Check sheet for the modelled part. Datum: model origin and axes. Units: mm. A direction names the side the tool comes from. Coordinates: 2 decimals unless noted, no trailing zeros. Order: outer loops, then holes, each group sorted by start corner. A loop starts at its lowest first (then second) coordinate and runs counter-clockwise, first axis right, second up. Notation, with made-up numbers: M 66,69 L 122,69 A31 ccw 122,102 Z; hole C -6,5 d8. An arc over 180 degrees is marked long. Answer in a Markdown table with one row per item. Add a question column.
from build123d import *

# Parameters (mm, degrees)
AUFSATZ_LINEAR_AUSTRAGEN1_DEPTH = 1566.7
SCHNITT_LINEAR_AUSTRAGEN1_REACH = 1704.359
FASE1_SIZE2                     = 30
FASE1_SIZE                      = 22
VERRUNDUNG1_R                   = 10
SKIZZE4_R                       = 14.488887394336269
AUFSATZ_LINEAR_AUSTRAGEN3_DEPTH = 30
AUFSATZ_LINEAR_AUSTRAGEN7_REACH = 1402.712
LINEARES_MUSTER2_COUNT          = 2
LINEARES_MUSTER2_PITCH          = 770.0000000000005


with BuildPart() as part:
    # Skizze1 → Aufsatz-Linear austragen1 (new body)
    with BuildSketch(Plane.XY):
        Polygon((650.3604764885325, 174.22108378429925), (650.3604764885325, 144.22108378429925), (227.86047648853256, 257.42961758644554), (72.86047648853256, 257.42961758644554), (-349.6395235114674, 144.22108378429914), (-349.6395235114674, 174.2210837842995), (72.86047648853253, 287.42961758644606), (227.8604764885318, 287.42961758644606), align=None)
    extrude(amount=AUFSATZ_LINEAR_AUSTRAGEN1_DEPTH)

    # Skizze2 → Schnitt-Linear austragen1 (cut, up to next)
    with BuildSketch(Plane(origin=(0, 287.42961758644606, 0), x_dir=(1, 0, 0), z_dir=(0, 1, 0)), mode=Mode.PRIVATE) as schnitt_linear_austragen1_sk1:
        Polygon((145.36047648853253, -360), (-289.47952351146745, -360.00000000000006), (-289.47952351146733, -1160.0000000000002), (145.36047648853264, -1160.0000000000005), align=None)
    schnitt_linear_austragen1_tool1 = extrude(schnitt_linear_austragen1_sk1.sketch, amount=-SCHNITT_LINEAR_AUSTRAGEN1_REACH, mode=Mode.PRIVATE) & part.part
    # Skizze2 → Schnitt-Linear austragen1 (cut, up to next)
    with BuildSketch(Plane(origin=(0, 287.42961758644606, 0), x_dir=(1, 0, 0), z_dir=(0, 1, 0)), mode=Mode.PRIVATE) as schnitt_linear_austragen1_sk2:
        Polygon((213.10047648853242, -373), (577.1204764885325, -372.99999999999994), (577.1204764885326, -847), (213.10047648853248, -847.0000000000001), align=None)
    schnitt_linear_austragen1_tool2 = extrude(schnitt_linear_austragen1_sk2.sketch, amount=-SCHNITT_LINEAR_AUSTRAGEN1_REACH, mode=Mode.PRIVATE) & part.part
    add(schnitt_linear_austragen1_tool1.solids().sort_by_distance((-72.059524, 287.429618, 760))[0], mode=Mode.SUBTRACT)
    add(schnitt_linear_austragen1_tool2.solids().sort_by_distance((395.110476, 287.429618, 610))[0], mode=Mode.SUBTRACT)

    # Fase1
    fase1_edges = [part.edges().sort_by_distance(p)[0] for p in [
        (-289.47952351146745, 190.34090720095548, 760.0000000000001),
    ]]
    fase1_side = [part.faces().sort_by_distance(p)[0] for p in [
        (-289.90453087503465, 190.22702682111037, 760.0000000000001),
    ]]
    chamfer(fase1_edges, length=FASE1_SIZE - 0.0001, length2=FASE1_SIZE2 - 0.0001, reference=fase1_side[0])  # a hair under: the kernel refuses the full size

    # Verrundung1
    verrundung1_edges = [part.edges().sort_by_distance(p)[0] for p in [
        (402.49047648853224, 240.6376501122001, 847),
    ]]
    fillet(verrundung1_edges, radius=VERRUNDUNG1_R)
    verrundung1_2_edges = [part.edges().sort_by_distance(p)[0] for p in [
        (577.1204764885325, 193.84568263795418, 610),
    ]]
    fillet(verrundung1_2_edges, radius=VERRUNDUNG1_R - 0.0001)  # a hair under: the kernel refuses the full size
    verrundung1_3_edges = [part.edges().sort_by_distance(p)[0] for p in [
        (402.4904764885322, 240.6376501122001, 373),
    ]]
    fillet(verrundung1_3_edges, radius=VERRUNDUNG1_R)

    # Skizze4 → Aufsatz-Linear austragen3 (add)
    with BuildSketch(Plane(origin=(-5.9234e-13, 0, 1160.0000000000005), x_dir=(-1, 0, -5.1e-16), z_dir=(5.1e-16, 0, -1))):
        with Locations(Location((-76.61047648853322, 273.43442705806245, 0), (0, 0, 105))):
            Circle(SKIZZE4_R)
    aufsatz_linear_austragen3 = extrude(amount=AUFSATZ_LINEAR_AUSTRAGEN3_DEPTH)

    # Aufsatz-Linear austragen7: up to this face of the body (flat: up to its plane)
    aufsatz_linear_austragen7_end = Plane(part.part.faces().sort_by_distance((-85.378398687, 228.495263502, 1160))[0])
    # Skizze6 → Aufsatz-Linear austragen7 (add, up to the picked face)
    with BuildSketch(Plane.XY.offset(360), mode=Mode.PRIVATE) as aufsatz_linear_austragen7_sk1:
        with BuildLine():
            Line((145.36047648853247, 287.42961758644606), (145.36047648853247, 257.42961758644554))
            Line((145.36047648853247, 257.42961758644554), (84.35616614086427, 257.42961758644554))
            Line((84.35616614086427, 257.42961758644554), (84.35616614086427, 261.189748632905))
            ThreePointArc((84.35616614086427, 261.189748632905), (89.30209346766217, 266.44509830768715), (91.09936388286874, 273.43442705806245))
            Line((91.09936388286874, 273.43442705806245), (109.11047648853247, 287.42961758644606))
            Line((109.11047648853247, 287.42961758644606), (145.36047648853247, 287.42961758644606))
        make_face()
    aufsatz_linear_austragen7_tool1 = split(extrude(aufsatz_linear_austragen7_sk1.sketch, amount=AUFSATZ_LINEAR_AUSTRAGEN7_REACH, mode=Mode.PRIVATE), bisect_by=aufsatz_linear_austragen7_end, keep=Keep.BOTH, mode=Mode.PRIVATE)
    add(aufsatz_linear_austragen7_tool1.solids().sort_by(Axis((118.992611, 271.244941, 360), (0, 0, 1)))[0])

    # Lineares Muster2: Aufsatz-Linear austragen3 ×2
    with Locations(*[(0, 0, -i * LINEARES_MUSTER2_PITCH) for i in range(1, LINEARES_MUSTER2_COUNT)]):
        add(aufsatz_linear_austragen3)


solid = part.part
1. Go/stop test with flat-tipped pins: pin 1 Ø15 at (y, z) = (267.5, 508.5) entering from +X; pin 2 Ø10 at (x, y) = (-119.5, 205.5) entering from +Z; pin 3 Ø3 at (x, z) = (-160, 270) entering from +Y; pin 4 Ø3 at (y, z) = (258.5, 616.5) entering from -X. Record where each tip stops, or that it passes through.
2. Set-up check for faces 1 (the flat face through (396, 223, 847)), 2 (the cylindrical face through (63.67, 279.95, 1145.21)), 3 (the flat face through (77, 273, 390)): record each of +Z, -Z, +X, -X, +Y, -Y from which the full face is reachable in a straight line by a thin tool's end or side.
3. Section check A-A on z = 1188.5. Enter the section's corners in (x, y).
4. Section check D-D on z = 548.5. State how many separate pieces and enclosed holes the cut face has, then the cut area to 3 significant figures.
5. Release check for a two-part mould opening along X. For faces 4 (the flat face through (77, 273, 1130)), 5 (the flat face through (-329.12, 179.72, 772.38)), 6 (the flat face through (442.068, 200.033, 946.461)) record: released by +X, released by -X, zero draft, split by the parting line, or undercut.
6. Section check C-C on x = -256. Enter the section's corners in (y, z), then the cut area to 3 significant figures.
7. Scan lines: line 1 (Z direction, x = 88, y = 277); line 2 (Y direction, x = 72, z = 107); line 3 (Z direction, x = 286, y = 252). Record each from-to range of solid material in increasing order.
Result sheet:
| question | item | result |
|---|---|---|
| 1 | pin 1 | x = 213.1 |
| 1 | pin 2 | z = 1566.7 |
| 1 | pin 3 | y = 225.44 |
| 1 | pin 4 | x = 84.36 |
| 2 | face 1 | +Y, -Y |
| 2 | face 2 | none |
| 2 | face 3 | -X, +Y |
| 3 | outline | M -349.64,144.22 L 72.86,257.43 L 227.86,257.43 L 650.36,144.22 L 650.36,174.22 L 227.86,287.43 L 72.86,287.43 L -349.64,174.22 Z |
| 4 | separate pieces | 3 |
| 4 | enclosed holes | 0 |
| 4 | area | 7,230 mm^2 |
| 5 | face 4 | zero draft |
| 5 | face 5 | released by -X |
| 5 | face 6 | undercut |
| 6 | outline | M 169.31,0 L 199.31,0 L 199.31,360 L 169.31,360 Z; M 169.31,1160 L 199.31,1160 L 199.31,1566.7 L 169.31,1566.7 Z |
| 6 | area | 23,000 mm^2 |
| 7 | line 1 | 0 to 390, 1130 to 1566.7 |
| 7 | line 2 | 257.2 to 287.2 |
| 7 | line 3 | 0 to 373, 847 to 1566.7 |
